Here's how the part is built. I have some questions about the finished solid (model axes, mm). Face numbers are marked on the shaded views. Give positions to 0.01 mm unless a question says otherwise; leave off trailing zeros. Write each loop counter-clockwise with the first axis right and the second up, starting at its lowest first coordinate (ties: lowest second). Pieces come first, ordered by that corner, then holes. Notation, with made-up numbers: (87, 59.25) - (93, 59.25) arc R17 cw to (93, 89.25) - close; hole circle Ø6 at (12.5, 41). An arc over 180 degrees is marked (long way). Use one line per item in the form item = value. Start each with the question number.
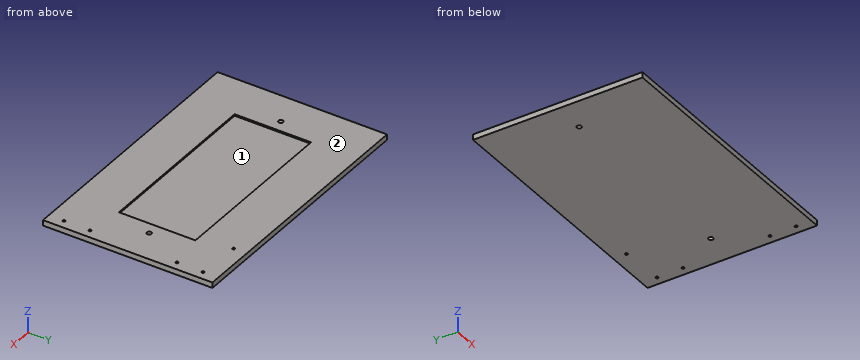
from build123d import *

# Parameters (mm, degrees)
F0_W     = 387.35
F0_H     = 247.65
F1_DEPTH = 8.001
F3_D     = 3.7973
F5_D     = 6.7564
F6_W     = 256.54
F6_H     = 111.76
F7_DEPTH = 2.286
F9_D     = 3.7973


with BuildPart() as f1:
    # F0 (on Top) → F1 (new body)
    with BuildSketch(Plane.XY):
        with Locations((193.675, 123.825)):
            Rectangle(F0_W, F0_H)
    extrude(amount=F1_DEPTH)

    # F3 (through all)
    with Locations(Plane.XY.offset(8.001)):
        with Locations((374.65, 225.425), (374.65, 187.325), (374.65, 60.325), (374.65, 22.225)):
            Hole(F3_D / 2)

    # F5 (through all)
    with Locations(Plane.XY.offset(8.001)):
        with Locations((47.625, 123.825), (339.725, 123.825)):
            Hole(F5_D / 2)

    # F6 (on face) → F7 (cut)
    with BuildSketch(Plane.XY.offset(8.001)):
        with Locations((193.675, 123.825)):
            Rectangle(F6_W, F6_H)
    extrude(amount=-F7_DEPTH, mode=Mode.SUBTRACT)

    # F9 (through all)
    with Locations(Plane.XY.offset(8.001)):
        with Locations((311.15, 228.6)):
            Hole(F9_D / 2)


solid = f1.part
1. For P1, Ø4, axis at x = 290, y = 157, coming from the +Z side (3 decimals), with a flat end and sliding along its axis, tell me the tip position at first contact or that it passes through.
2. I want a section at B-B, the plane y = 169. List the corners of the cut face in (x, z) for me (3 decimals), then the cut area to 3 significant figures.
3. I want a section at A-A, the plane x = 234. List the corners of the cut face in (y, z) for me (3 decimals).
4. Please list where these lines run through material, in increasing order: line 1 (Y direction, x = 374.65, z = 6.5); line 2 (Y direction, x = 135, z = 7.25) (3 decimals); line 3 (X direction, y = 106, z = 7.5) (3 decimals).
5. We'd pull the mould along Y, two halves only. Please class the marked faces 1 and 2: pulls with the +Y half, pulls with the -Y half, needs draft (parallel to the pull), parting line crosses it, or undercut.
Result sheet:
q1.P1 = 5.715
q2.outline = (0, 0) - (387.35, 0) - (387.35, 8.001) - (321.945, 8.001) - (321.945, 5.715) - (65.405, 5.715) - (65.405, 8.001) - (0, 8.001) - close
q2.area = 2,510 mm2
q3.outline = (0, 0) - (247.65, 0) - (247.65, 8.001) - (179.705, 8.001) - (179.705, 5.715) - (67.945, 5.715) - (67.945, 8.001) - (0, 8.001) - close
q4.line_1 = 0 to 20.33, 24.12 to 58.43, 62.22 to 185.43, 189.22 to 223.53, 227.32 to 247.65
q4.line_2 = 0 to 67.945, 179.705 to 247.65
q4.line_3 = 0 to 65.405, 321.945 to 387.35
q5.face_1 = undercut
q5.face_2 = needs draft
